from build123d import *

# Parameters (mm, degrees)
F1_DEPTH = 60
F2_R     = 5
F3_SIZE  = 5
F5_R     = 21.846127
F6_DEPTH = 30


with BuildPart() as f1:
    # F0 (on Front) → F1 (new body)
    with BuildSketch(Plane.XZ):
        with BuildLine():
            Line((49.28327, 51.693205), (-35.71673, 51.693205))
            ThreePointArc((-35.71673, 51.693205), (-46.323332, 47.299807), (-50.71673, 36.693205))
            Line((-50.71673, 36.693205), (-50.71673, -48.306795))
            Line((-50.71673, -48.306795), (34.28327, -48.306795))
            ThreePointArc((34.28327, -48.306795), (44.889872, -43.913397), (49.28327, -33.306795))
            Line((49.28327, -33.306795), (49.28327, 51.693205))
        make_face()
    extrude(amount=F1_DEPTH)

    # F2
    f2_edges = [f1.edges().sort_by_distance(p)[0] for p in [
        (49.28327, 0, 9.193205),
        (6.78327, 0, 51.693205),
        (-46.323332, 0, 47.299807),
        (-50.71673, 0, -5.806795),
        (-8.21673, 0, -48.306795),
        (44.889872, 0, -43.913397),
    ]]
    fillet(f2_edges, radius=F2_R)

    # F3
    f3_edges = [f1.edges().sort_by_distance(p)[0] for p in [
        (49.28327, -60, 9.193205),
        (6.78327, -60, 51.693205),
        (-46.323332, -60, 47.299807),
        (-50.71673, -60, -5.806795),
        (-8.21673, -60, -48.306795),
        (44.889872, -60, -43.913397),
    ]]
    chamfer(f3_edges, length=F3_SIZE)

    # F5 (on face) → F6 (cut)
    with BuildSketch(Plane.XZ.offset(60)):
        Circle(F5_R)
    extrude(amount=-F6_DEPTH, mode=Mode.SUBTRACT)


solid = f1.part
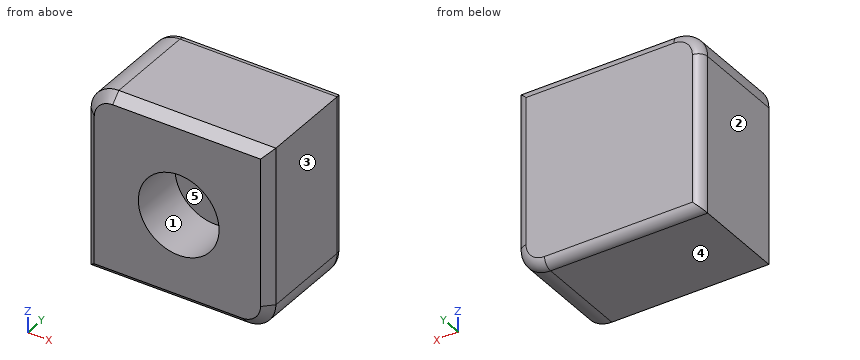
Check sheet for the modelled part. Datum: model origin and axes. Units: mm. Face numbers are marked on the shaded views. A direction names the side the tool comes from. Give positions to 0.01 mm unless a question says otherwise; leave off trailing zeros. Loops run counter-clockwise (first coordinate to the right, second up) from the corner with the lowest first, then second, coordinate; pieces in that order, holes last. Notation, with made-up numbers: M 54,82.5 L 71,82.5 A15 cw 71,107.5 Z; hole C -15,-1.5 d7. An arc over 180 degrees is marked long. Answer as a JSON object with one key per item and string values. Group by question number.
Q1. Material ranges on line 1 along Z through (x, y) = (0, -52); line 2 along Y through (x, z) = (-10.5, 16.5); line 3 along Z through (x, y) = (16.5, -39.5), recorded low to high. Write a range as [from, to].
Q2. Access from +Z, -Z, +X, -X, +Y, -Y to the whole of each face (thin tool, end or side, straight path). Record for the marked faces 1 and 2.
Q3. Cross-section at A-A on y = -39. Record the cut outline in (x, z), then the cut area to 3 significant figures.
Q4. Cross-section at C-C on x = 0. Record the cut outline in (y, z), then the cut area to 3 significant figures.
Q5. Cross-section at B-B on z = 0. Record the cut outline in (x, y).
Q6. Release check for a two-part mould opening along Z. For the marked faces 3, 4 and 5 record: released by +Z, released by -Z, zero draft, split by the parting line, or undercut.
Evaluation:
{
 "1": {"line 1": "z = [-48.31, -21.85], [21.85, 51.69]", "line 2": "y = [-30, 0]", "line 3": "z = [-48.31, -14.32], [14.32, 51.69]"},
 "2": {"face 1": "-Y", "face 2": "+Z, -Z, -X, +Y, -Y"},
 "3": {"outline": "M -50.72,-48.31 L 34.28,-48.31 A15 ccw 49.28,-33.31 L 49.28,51.69 L -35.72,51.69 A15 ccw -50.72,36.69 Z; hole C 0,0 d43.69", "area": "8,400 mm2"},
 "4": {"outline": "M -60,-43.31 L -55,-48.31 L -5,-48.31 A5 ccw 0,-43.31 L 0,46.69 A5 ccw -5,51.69 L -55,51.69 L -60,46.69 L -60,21.85 L -30,21.85 L -30,-21.85 L -60,-21.85 Z", "area": "4,650 mm2"},
 "5": {"outline": "M -50.72,-55 L -45.72,-60 L -21.85,-60 L -21.85,-30 L 21.85,-30 L 21.85,-60 L 44.28,-60 L 49.28,-55 L 49.28,-5 A5 ccw 44.28,0 L -45.72,0 A5 ccw -50.72,-5 Z"},
 "6": {"face 3": "zero draft", "face 4": "released by -Z", "face 5": "undercut"}
}
